Job drawing, mm, ordinate dimensions from the low corner. One solid piece. A direction names the side the tool comes from. Give positions to 0.01 mm unless a question says otherwise; leave off trailing zeros. Write each loop counter-clockwise with the first axis right and the second up, starting at its lowest first coordinate (ties: lowest second). Pieces come first, ordered by that corner, then holes. Notation, with made-up numbers: M 61,36 L 106,36 A27 ccw 106,60 Z; hole C 1.5,63 d2. An arc over 180 degrees is marked long. Answer as CSV lines item,"result". Start each with the question number.
Item 1: 3-axis set-ups, long thin cutter, end or side, ignore diameter. For the marked faces 1, 2 and 3: which of +Z, -Z, +X, -X, +Y, -Y reach the whole face in a straight line?
Item 2: Band-saw the part on B-B, the plane z = 19.5. List the corners of the cut face in (x, y), then the cut area to 3 significant figures.
Item 3: Wall check: L1, parallel to Y at x = 19.6, z = 36; L2, parallel to X at y = 1.25, z = 5.5; L3, parallel to Y at x = 12.6, z = 36.4. Give the ranges that are in metal, low to high. Write a range as from..to.
Item 4: Band-saw the part on A-A, the plane x = 40.6. Count the separate pieces of the cut face and the enclosed holes in it, then the cut area to 3 significant figures.
Item 5: Pin check, flat tips, straight feed: pin 1 (2.5 mm diameter, centred on x = 54, y = 1, fed in from +Z); pin 2 (4 mm diameter, centred on x = 19.6, y = 13, fed in from -Z); pin 3 (0.7 mm diameter, centred on y = 1, z = 5.5, fed in from -X); pin 4 (4 mm diameter, centred on x = 9.5, z = 19.5, fed in from +Y). Stop position of each tip, or through.
Item 6: Band-saw the part on D-D, the plane z = 5.5. List the corners of the cut face in (x, y).
Item 7: Band-saw the part on C-C, the plane y = 20. List the corners of the cut face in (x, z), then the cut area to 3 significant figures.
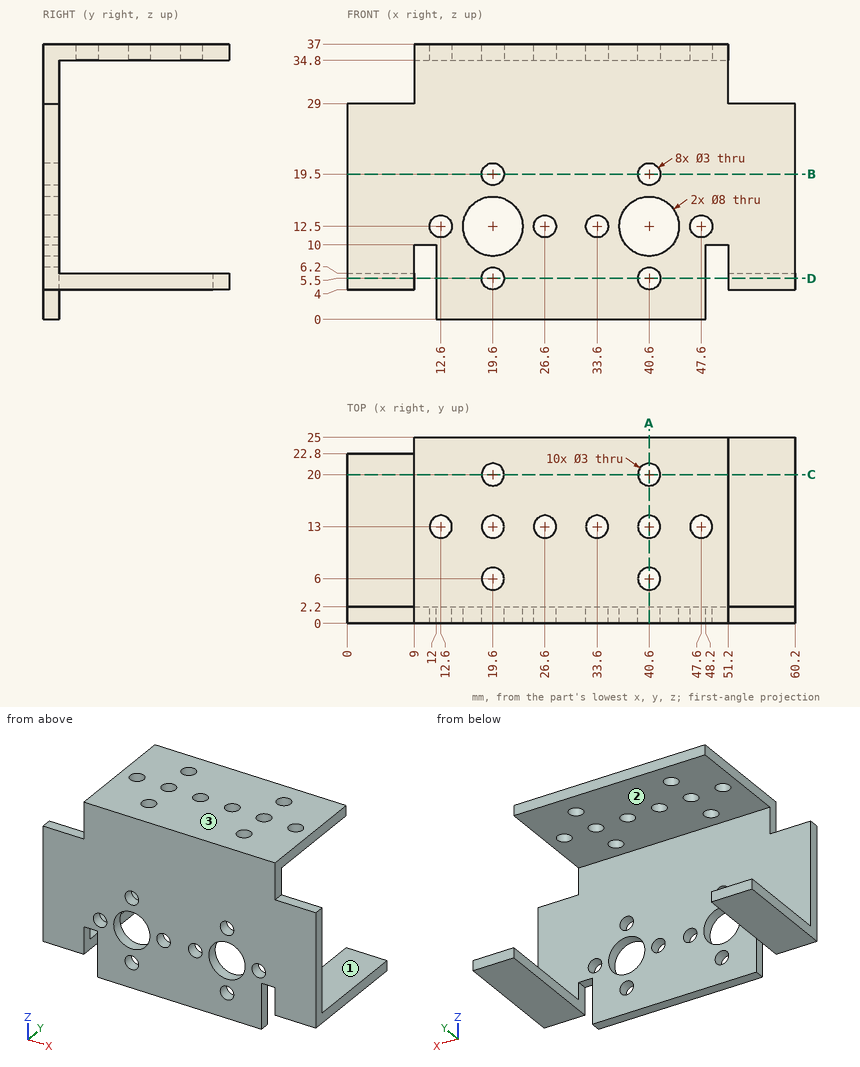
Output:
1,face 1,"+Z, +X, -X, +Y"
1,face 2,"-Z, +X, -X, +Y"
1,face 3,"+Z, +X, -X, +Y, -Y"
2,outline,"M 0,0 L 18.1,0 L 18.1,2.2 L 0,2.2 Z; M 21.1,0 L 39.1,0 L 39.1,2.2 L 21.1,2.2 Z; M 42.1,0 L 60.2,0 L 60.2,2.2 L 42.1,2.2 Z"
2,area,"119 mm²"
3,L1,"0..4.5, 7.5..11.5, 14.5..18.5, 21.5..25"
3,L2,"0..9, 12..18.1, 21.1..39.1, 42.1..48.2, 51.2..60.2"
3,L3,"0..11.5, 14.5..25"
4,separate pieces,"7"
4,enclosed holes,"0"
4,area,"81.0 mm²"
5,pin 1,"z = 29"
5,pin 2,"z = 34.8"
5,pin 3,"x = 0"
5,pin 4,"y = 2.2"
6,outline,"M 0,0 L 9,0 L 9,22.8 L 0,22.8 Z; M 12,0 L 18.1,0 L 18.1,2.2 L 12,2.2 Z; M 21.1,0 L 39.1,0 L 39.1,2.2 L 21.1,2.2 Z; M 42.1,0 L 48.2,0 L 48.2,2.2 L 42.1,2.2 Z; M 51.2,0 L 60.2,0 L 60.2,25 L 51.2,25 Z"
7,outline,"M 0,4 L 9,4 L 9,6.2 L 0,6.2 Z; M 9,34.8 L 18.1,34.8 L 18.1,37 L 9,37 Z; M 21.1,34.8 L 39.1,34.8 L 39.1,37 L 21.1,37 Z; M 42.1,34.8 L 51.2,34.8 L 51.2,37 L 42.1,37 Z; M 51.2,4 L 60.2,4 L 60.2,6.2 L 51.2,6.2 Z"
7,area,"119 mm²"
